Build history of the part. All positions in model axes, mm. A direction names the side the tool comes from. Give positions to 0.01 mm unless a question says otherwise; leave off trailing zeros. Order: outer loops, then holes, each group sorted by start corner. A loop starts at its lowest first (then second) coordinate and runs counter-clockwise, first axis right, second up. Notation, with made-up numbers: (26, 17) -> (56, 17) arc R29 cw to (56, 56) -> close; hole circle Ø8 at (49, -15.5). An arc over 180 degrees is marked (long way). Use a Markdown table: item, result. Add a question column.
```python
from build123d import *

# Parameters (mm, degrees)
SKETCH1_R                = 57.15
BOSS_EXTRUDE1_DEPTH      = 2
SKETCH2_R                = 53.75
SKETCH2_R_2              = 51.75
BOSS_EXTRUDE2_DEPTH      = 16.25
CUT_EXTRUDE1_DEPTH       = 16.25
CUT_EXTRUDE2_DEPTH       = 6.8
BOSS_EXTRUDE5_DEPTH      = 16.25
CUT_EXTRUDE3_DEPTH       = 7.6
SKETCH9_W                = 2
SKETCH9_H                = 2
SKETCH9_H_2              = 12.25
CUT_EXTRUDE4_DEPTH       = 58.15
CUT_EXTRUDE5_DEPTH       = 16.25
SKETCH12_W               = 4.25
SKETCH12_H               = 14.29
SKETCH12_R               = 57.15
BOSS_EXTRUDE7_DEPTH      = 2
BOSS_EXTRUDE8_DEPTH      = 13.9
BOSS_EXTRUDE9_DEPTH      = 2
BOSS_EXTRUDE9_DEPTH_BACK = 2
BOSS_EXTRUDE10_DEPTH     = 13.9


with BuildPart() as part:
    # Sketch1 → Boss-Extrude1 (new body)
    with BuildSketch(Plane(origin=(0, 0, 0), x_dir=(1, 0, 0), z_dir=(0, 1, 0))):
        Circle(SKETCH1_R)
    extrude(amount=BOSS_EXTRUDE1_DEPTH)

    # Sketch2 → Boss-Extrude2 (add)
    with BuildSketch(Plane(origin=(0, 2, 0), x_dir=(1, 0, 0), z_dir=(0, 1, 0))):
        Circle(SKETCH2_R)
        Circle(SKETCH2_R_2, mode=Mode.SUBTRACT)
    extrude(amount=BOSS_EXTRUDE2_DEPTH)

    # Sketch4 → Cut-Extrude1 (cut)
    with BuildSketch(Plane(origin=(0, 18.25, 0), x_dir=(1, 0, 0), z_dir=(0, 1, 0))):
        with BuildLine():
            ThreePointArc((51.75, 0), (51.741714453, -0.926005111), (51.716860465, -1.851713701))
            ThreePointArc((51.716860465, -1.851713701), (52.606544101, -2.501001521), (53.679651163, -2.749100042))
            ThreePointArc((53.679651163, -2.749100042), (53.732409912, -1.375), (53.75, 0))
            ThreePointArc((53.75, 0), (53.732409912, 1.375), (53.679651163, 2.749100042))
            ThreePointArc((53.679651163, 2.749100042), (52.606544101, 2.501001521), (51.716860465, 1.851713701))
            ThreePointArc((51.716860465, 1.851713701), (51.741714453, 0.926005111), (51.75, 0))
        make_face()
        with BuildLine():
            ThreePointArc((-51.716860465, 1.851713701), (-51.75, 0), (-51.716860465, -1.851713701))
            ThreePointArc((-51.716860465, -1.851713701), (-52.606544101, -2.501001521), (-53.679651163, -2.749100042))
            ThreePointArc((-53.679651163, -2.749100042), (-53.75, 0), (-53.679651163, 2.749100042))
            ThreePointArc((-53.679651163, 2.749100042), (-52.606544101, 2.501001521), (-51.716860465, 1.851713701))
        make_face()
    extrude(amount=-CUT_EXTRUDE1_DEPTH, mode=Mode.SUBTRACT)

    # Sketch5 → Cut-Extrude2 (cut)
    with BuildSketch(Plane(origin=(0, 18.25, 0), x_dir=(1, 0, 0), z_dir=(0, 1, 0))):
        with BuildLine():
            Line((0, -53.75), (0, -51.75))
            ThreePointArc((0, -51.75), (-1.500631048, -51.728237999), (-3, -51.662970298))
            Line((-3, -51.662970298), (-3, -53.666213766))
            ThreePointArc((-3, -53.666213766), (-1.500584897, -53.729049358), (0, -53.75))
        make_face()
        with BuildLine():
            ThreePointArc((3, -51.662970298), (1.500631048, -51.728237999), (0, -51.75))
            Line((0, -51.75), (0, -53.75))
            ThreePointArc((0, -53.75), (1.500584897, -53.729049358), (3, -53.666213766))
            Line((3, -53.666213766), (3, -51.662970298))
        make_face()
    extrude(amount=-CUT_EXTRUDE2_DEPTH, mode=Mode.SUBTRACT)

    # Sketch7 → Boss-Extrude5 (add)
    with BuildSketch(Plane(origin=(0, 2, 0), x_dir=(1, 0, 0), z_dir=(0, 1, 0))):
        with BuildLine():
            Line((2.4, -54.571141496), (2.4, -57.099584062))
            ThreePointArc((2.4, -57.099584062), (0, -57.15), (-2.4, -57.099584062))
            Line((-2.4, -57.099584062), (-2.4, -54.571141496))
            ThreePointArc((-2.4, -54.571141496), (0, -54.623891148), (2.4, -54.571141496))
        make_face()
    extrude(amount=BOSS_EXTRUDE5_DEPTH)

    # Sketch8 → Cut-Extrude3 (cut)
    with BuildSketch(Plane.XY.offset(57.15)):
        with BuildLine():
            Line((2.4, 11.75), (2.4, 13.55))
            ThreePointArc((2.4, 13.55), (0, 14.75), (-2.4, 13.55))
            Line((-2.4, 13.55), (-2.4, 11.75))
            Line((-2.4, 11.75), (2.4, 11.75))
        make_face()
        with BuildLine():
            Line((2.4, 9.95), (2.4, 11.75))
            Line((2.4, 11.75), (-2.4, 11.75))
            Line((-2.4, 11.75), (-2.4, 9.95))
            ThreePointArc((-2.4, 9.95), (0, 8.75), (2.4, 9.95))
        make_face()
        with BuildLine():
            Line((2.4, 11.75), (2.4, 13.55))
            ThreePointArc((2.4, 13.55), (0, 14.75), (-2.4, 13.55))
            Line((-2.4, 13.55), (-2.4, 11.75))
            Line((-2.4, 11.75), (2.4, 11.75))
        make_face()
        with BuildLine():
            Line((2.4, 9.95), (2.4, 11.75))
            Line((2.4, 11.75), (-2.4, 11.75))
            Line((-2.4, 11.75), (-2.4, 9.95))
            ThreePointArc((-2.4, 9.95), (0, 8.75), (2.4, 9.95))
        make_face()
        with BuildLine():
            Line((2.4, 13.55), (2.4, 18.25))
            Line((2.4, 18.25), (-2.4, 18.25))
            Line((-2.4, 18.25), (-2.4, 13.55))
            ThreePointArc((-2.4, 13.55), (0, 14.75), (2.4, 13.55))
        make_face()
        with BuildLine():
            ThreePointArc((3, 11.75), (2.846049894, 12.698683298), (2.4, 13.55))
            Line((2.4, 13.55), (2.4, 11.75))
            Line((2.4, 11.75), (2.4, 9.95))
            ThreePointArc((2.4, 9.95), (2.846049894, 10.801316702), (3, 11.75))
        make_face()
        with BuildLine():
            Line((-2.4, 11.75), (-2.4, 13.55))
            ThreePointArc((-2.4, 13.55), (-3, 11.75), (-2.4, 9.95))
            Line((-2.4, 9.95), (-2.4, 11.75))
        make_face()
    extrude(amount=-CUT_EXTRUDE3_DEPTH, mode=Mode.SUBTRACT)

    # Sketch9 → Cut-Extrude4 (cut, through all)
    with BuildSketch(Plane.XY):
        with Locations((0, 5)):
            Rectangle(SKETCH9_W, SKETCH9_H)
        with Locations((0, 12.125)):
            Rectangle(SKETCH9_W, SKETCH9_H_2)
    extrude(amount=-CUT_EXTRUDE4_DEPTH, mode=Mode.SUBTRACT)

    # Sketch11 → Cut-Extrude5 (cut)
    with BuildSketch(Plane(origin=(0, 18.25, 0), x_dir=(1, 0, 0), z_dir=(0, 1, 0))):
        with BuildLine():
            Line((7.9, -53.166272203), (7.9, -51.143450216))
            ThreePointArc((7.9, -51.143450216), (5.456186881, -51.461563567), (3, -51.662970298))
            Line((3, -51.662970298), (3, -53.666213766))
            ThreePointArc((3, -53.666213766), (5.455729593, -53.472399559), (7.9, -53.166272203))
        make_face()
        with BuildLine():
            ThreePointArc((-3, -51.662970298), (-5.456186881, -51.461563567), (-7.9, -51.143450216))
            Line((-7.9, -51.143450216), (-7.9, -53.166272203))
            ThreePointArc((-7.9, -53.166272203), (-5.455729593, -53.472399559), (-3, -53.666213766))
            Line((-3, -53.666213766), (-3, -51.662970298))
        make_face()
        with BuildLine():
            Line((7.9, -51.143450216), (7.9, -49.368739918))
            Line((7.9, -49.368739918), (-7.9, -49.368739918))
            Line((-7.9, -49.368739918), (-7.9, -51.143450216))
            ThreePointArc((-7.9, -51.143450216), (-5.456186881, -51.461563567), (-3, -51.662970298))
            Line((-3, -51.662970298), (-3, -53.666213766))
            ThreePointArc((-3, -53.666213766), (-5.455729593, -53.472399559), (-7.9, -53.166272203))
            Line((-7.9, -53.166272203), (-7.9, -53.957200677))
            Line((-7.9, -53.957200677), (7.9, -53.957200677))
            Line((7.9, -53.957200677), (7.9, -53.166272203))
            ThreePointArc((7.9, -53.166272203), (5.455729593, -53.472399559), (3, -53.666213766))
            Line((3, -53.666213766), (3, -51.662970298))
            ThreePointArc((3, -51.662970298), (5.456186881, -51.461563567), (7.9, -51.143450216))
        make_face()
    extrude(amount=-CUT_EXTRUDE5_DEPTH, mode=Mode.SUBTRACT)

    # Sketch12 → Boss-Extrude7 (add)
    with BuildSketch(Plane.XZ):
        with Locations((2.125, 64.295)):
            Rectangle(SKETCH12_W, SKETCH12_H)
        with Locations((-2.125, 64.295)):
            Rectangle(SKETCH12_W, SKETCH12_H)
        with BuildLine():
            Line((4.25, 57.15), (0, 57.15))
            ThreePointArc((0, 57.15), (2.126472541, 57.110424745), (4.25, 56.991753789))
            Line((4.25, 56.991753789), (4.25, 57.15))
        make_face()
        with BuildLine():
            ThreePointArc((-4.25, 56.991753789), (-2.126472541, 57.110424745), (0, 57.15))
            Line((0, 57.15), (-4.25, 57.15))
            Line((-4.25, 57.15), (-4.25, 56.991753789))
        make_face()
        with Locations((2.125, -64.295)):
            Rectangle(SKETCH12_W, SKETCH12_H)
        with Locations((-2.125, -64.295)):
            Rectangle(SKETCH12_W, SKETCH12_H)
        with BuildLine():
            ThreePointArc((0, -57.15), (-2.126472541, -57.110424745), (-4.25, -56.991753789))
            Line((-4.25, -56.991753789), (-4.25, -57.15))
            Line((-4.25, -57.15), (0, -57.15))
        make_face()
        with BuildLine():
            Line((4.25, -57.15), (4.25, -56.991753789))
            ThreePointArc((4.25, -56.991753789), (2.126472541, -57.110424745), (0, -57.15))
            Line((0, -57.15), (4.25, -57.15))
        make_face()
        Circle(SKETCH12_R)
    extrude(amount=-BOSS_EXTRUDE7_DEPTH)

    # Sketch13 → Boss-Extrude8 (add)
    with BuildSketch(Plane.XY.offset(71.44)):
        with BuildLine():
            Line((-3, 11.75), (-4.25, 11.75))
            Line((-4.25, 11.75), (-4.25, 2))
            Line((-4.25, 2), (4.25, 2))
            Line((4.25, 2), (4.25, 11.75))
            Line((4.25, 11.75), (3, 11.75))
            ThreePointArc((3, 11.75), (0, 8.75), (-3, 11.75))
        make_face()
    extrude(amount=-BOSS_EXTRUDE8_DEPTH)

    # Sketch14 → Boss-Extrude9 (add, two sides)
    with BuildSketch(Plane.XY.offset(57.15)) as boss_extrude9_sk:
        with BuildLine():
            Line((-2.4, 2), (2.4, 2))
            Line((2.4, 2), (2.4, 9.95))
            ThreePointArc((2.4, 9.95), (0, 8.75), (-2.4, 9.95))
            Line((-2.4, 9.95), (-2.4, 2))
        make_face()
    extrude(amount=BOSS_EXTRUDE9_DEPTH)
    extrude(boss_extrude9_sk.sketch, amount=-BOSS_EXTRUDE9_DEPTH_BACK)

    # Sketch15 → Boss-Extrude10 (add)
    with BuildSketch(Plane(origin=(0, 0, -71.44), x_dir=(-1, 0, 0), z_dir=(0, 0, -1))):
        with BuildLine():
            Line((-1.5, 11.75), (-4.25, 11.75))
            Line((-4.25, 11.75), (-4.25, 0))
            Line((-4.25, 0), (4.25, 0))
            Line((4.25, 0), (4.25, 11.75))
            Line((4.25, 11.75), (1.5, 11.75))
            ThreePointArc((1.5, 11.75), (0, 10.25), (-1.5, 11.75))
        make_face()
    extrude(amount=-BOSS_EXTRUDE10_DEPTH)


solid = part.part
```
(1) Wall check: probe 1 along Y at (x, z) = (-13, 49.5); probe 2 along X at (y, z) = (13, 14); probe 3 along Z at (x, y) = (20.5, 7.25). Give the ranges that are in metal, low to high.
(2) Pin check, flat tips, straight feed: pin 1 Ø1 at (x, y) = (12, 13.5) entering from +Z; pin 2 Ø3.5 at (y, z) = (3, 66.5) entering from +X; pin 3 Ø6 at (y, z) = (3.5, -65) entering from -X; pin 4 Ø3 at (x, z) = (34.5, 42.5) entering from -Y. Stop position of each tip, or through.
(3) Tool access for faces 1 (the face through (0.07, 8.75, 63.12)), 2 (the face through (4.25, 6, -64)), 3 (the face through (-40.138, 10.011, 35.749)), 4 (the face through (38.3, 10, 34.8)), 5 (the face through (-2.4, 6, 56)): list every direction of +Z, -Z, +X, -X, +Y, -Y with a clear straight run to the whole face (end or side of a thin tool).
(4) Band-saw the part on C-C on x = 28. Give the cut face in (y, z).
(5) Band-saw the part on A-A on y = 15.75. Give the cut face in (x, z).
(6) Band-saw the part on B-B on z = 12.5. Give the cut face in (x, y).
(7) Mould opens along X. For faces 6 (the face through (-4.25, 6, 64)), 7 (the face through (4.25, 6, 64)), 8 (the face through (-0.03, 10.25, -64.59)) say: released by +X, released by -X, zero draft, split by the parting line, or undercut.
Response:
| question | item | result |
|---|---|---|
| 1 | probe 1 | y = 0 to 2 |
| 1 | probe 2 | x = -51.89 to -49.82, 49.82 to 51.89 |
| 1 | probe 3 | z = -49.69 to -47.52, 47.52 to 49.69 |
| 2 | pin 1 | stops at z = 52.51 |
| 2 | pin 2 | stops at x = 4.25 |
| 2 | pin 3 | stops at x = -4.25 |
| 2 | pin 4 | stops at y = 0 |
| 3 | face 1 | +Z, +Y |
| 3 | face 2 | -Z, +X, +Y, -Y |
| 3 | face 3 | +Z, -X, +Y |
| 3 | face 4 | +Y |
| 3 | face 5 | -X, +Y |
| 4 | outline | (0, -49.82) -> (2, -49.82) -> (2, -45.88) -> (18.25, -45.88) -> (18.25, -43.52) -> (2, -43.52) -> (2, 43.52) -> (18.25, 43.52) -> (18.25, 45.88) -> (2, 45.88) -> (2, 49.82) -> (0, 49.82) -> close |
| 5 | outline | (-53.68, -2.75) arc R53.75 ccw to (-1, -53.74) -> (-1, -51.74) arc R51.75 cw to (-51.72, -1.85) arc R2.75 cw to start; (-53.68, 2.75) arc R2.75 cw to (-51.72, 1.85) arc R51.75 cw to (-7.9, 51.14) -> (-7.9, 53.17) arc R53.75 ccw to start; (1, -53.74) arc R53.75 ccw to (53.68, -2.75) arc R2.75 cw to (51.72, -1.85) arc R51.75 cw to (1, -51.74) -> close; (7.9, 51.14) arc R51.75 cw to (51.72, 1.85) arc R2.75 cw to (53.68, 2.75) arc R53.75 ccw to (7.9, 53.17) -> close |
| 6 | outline | (-55.77, 0) -> (55.77, 0) -> (55.77, 2) -> (52.28, 2) -> (52.28, 18.25) -> (50.22, 18.25) -> (50.22, 2) -> (-50.22, 2) -> (-50.22, 18.25) -> (-52.28, 18.25) -> (-52.28, 2) -> (-55.77, 2) -> close |
| 7 | face 6 | released by -X |
| 7 | face 7 | released by +X |
| 7 | face 8 | undercut |
